Design review of the part built by this model. Coordinates are the model's own, in mm. A direction names the side the tool comes from. Round coordinates to 2 decimals unless told otherwise and drop trailing zeros. Loops run counter-clockwise (first coordinate to the right, second up) from the corner with the lowest first, then second, coordinate; pieces in that order, holes last. Notation, with made-up numbers: (33.25, -34) - (38.25, -34) arc R20 cw to (38.25, -14) - close; hole circle Ø1 at (-3, -26). An arc over 180 degrees is marked (long way). Return JSON: item names as keys, results as strings. Group by question number.
from build123d import *

# Parameters (mm, degrees)
SKETCH026_R     = 5
PAD015_DEPTH    = 0.5
SKETCH027_R     = 3
PAD016_DEPTH    = 3
FILLET003_R     = 1
SKETCH028_R     = 2.5
POCKET011_DEPTH = 1
FILLET004_R     = 0.6


with BuildPart() as part:
    # Sketch026 (on XY_Plane005 of Origin010) → Pad015 (new body)
    with BuildSketch(Plane.XY):
        Circle(SKETCH026_R)
    extrude(amount=PAD015_DEPTH)

    # Sketch027 (on Face3 of Pad015) → Pad016 (join)
    with BuildSketch(Plane.XY.offset(0.5)):
        Circle(SKETCH027_R)
    extrude(amount=PAD016_DEPTH)

    # Fillet003
    fillet003_edges = [part.edges().sort_by_distance(p)[0] for p in [
        (-3, 0, 3.5),
    ]]
    fillet(fillet003_edges, radius=FILLET003_R)

    # Sketch028 → Pocket011 (cut)
    with BuildSketch(Plane.XY):
        Circle(SKETCH028_R)
    extrude(amount=POCKET011_DEPTH, mode=Mode.SUBTRACT)

    # Fillet004
    fillet004_edges = [part.edges().sort_by_distance(p)[0] for p in [
        (-2.5, 0, 1),
    ]]
    fillet(fillet004_edges, radius=FILLET004_R)


solid = part.part
Q1. Insertion check: pin 1 Ø1.1 at (x, y) = (-0.5, -1) entering from -Z; pin 2 Ø1.5 at (y, z) = (-3.5, 1) entering from +X; pin 3 Ø2 at (y, z) = (-3, 2) entering from +X. Each pin has a flat end and moves straight along its axis. Give the tip position at first contact, or say it passes through.
Q2. Add section C-C, the plane z = 1.8. State the section outline as (x, y) points.
Q3. Add section D-D, the plane y = -3.5. State the section outline as (x, z) points, plus the area to 3 significant figures.
Q4. Tool access review of faces 1 (the cylindrical face through (-3, 0, 1)), 2 (the flat face through (0, 0, 3.5)), 3 (the cylindrical face through (-0.54, -2.44, 0.2)): name each direction out of +Z, -Z, +X, -X, +Y, -Y from which nothing blocks a thin tool from reaching the whole face with its end or side.
Q5. Add section A-A, the plane y = 0. State the section outline as (x, z) points.
Q6. Draft analysis for pull direction Y (two halves, no side actions). For faces 4 (the cylindrical face through (-1.08, -4.88, 0.25)), 5 (the flat face through (-0.1, -3.3, 0.5)), 6 (the flat face through (0, 0, 1)), state which applies: pulls with the +Y half, pulls with the -Y half, needs draft (parallel to the pull), parting line crosses it, or undercut.
Q7. For line 1 (Y direction, x = 0, z = 0.35); line 2 (Z direction, x = 3.5, y = 0.25); line 3 (Z direction, x = 0.25, y = -1.5), list the stretches that pass through material, from the lowest coordinate up.
Evaluation:
{
 "1": {"pin 1": "z = 1", "pin 2": "x = 4.04", "pin 3": "x = 2.24"},
 "2": {"outline": "circle Ø6 at (0, 0)"},
 "3": {"outline": "(-3.57, 0) - (3.57, 0) - (3.57, 0.5) - (-3.57, 0.5) - close", "area": "3.57 mm²"},
 "4": {"face 1": "+Z", "face 2": "+Z, +X, -X, +Y, -Y", "face 3": "-Z"},
 "5": {"outline": "(-5, 0) - (-2.5, 0) - (-2.5, 0.4) arc R0.6 cw to (-1.9, 1) - (1.9, 1) arc R0.6 cw to (2.5, 0.4) - (2.5, 0) - (5, 0) - (5, 0.5) - (3, 0.5) - (3, 2.5) arc R1 ccw to (2, 3.5) - (-2, 3.5) arc R1 ccw to (-3, 2.5) - (-3, 0.5) - (-5, 0.5) - close"},
 "6": {"face 4": "parting line crosses it", "face 5": "needs draft", "face 6": "undercut"},
 "7": {"line 1": "-5 to -2.5, 2.5 to 5", "line 2": "0 to 0.5", "line 3": "1 to 3.5"}
}
